```python
from build123d import *

# Parameters (mm, degrees)
F1_DEPTH = 3.5
F2_R     = 1.6
F3_DEPTH = 3.501


with BuildPart() as f1:
    # F0 (on Top) → F1 (new body)
    with BuildSketch(Plane.XY):
        with BuildLine():
            ThreePointArc((20, 4), (16, 0), (20, -4))
            Line((20, -4), (20, 4))
        make_face()
        with BuildLine():
            Line((-20, -4), (20, -4))
            ThreePointArc((20, -4), (16, 0), (20, 4))
            Line((20, 4), (-20, 4))
            ThreePointArc((-20, 4), (-17.1715728753, 2.8284271247), (-16, 0))
            ThreePointArc((-16, 0), (-17.1715728753, -2.8284271247), (-20, -4))
        make_face()
        with BuildLine():
            Line((20, 4), (20, -4))
            ThreePointArc((20, -4), (22.8284271247, -2.8284271247), (24, 0))
            ThreePointArc((24, 0), (22.8284271247, 2.8284271247), (20, 4))
        make_face()
        with BuildLine():
            ThreePointArc((-20, 4), (-24, 0), (-20, -4))
            Line((-20, -4), (-20, 4))
        make_face()
        with BuildLine():
            Line((-20, 4), (-20, -4))
            ThreePointArc((-20, -4), (-17.1715728753, -2.8284271247), (-16, 0))
            ThreePointArc((-16, 0), (-17.1715728753, 2.8284271247), (-20, 4))
        make_face()
    extrude(amount=F1_DEPTH)

    # F2 (on face) → F3 (cut, through all)
    with BuildSketch(Plane.XY.offset(3.5)):
        with BuildLine():
            ThreePointArc((-20, 1.6), (-21.6, 0), (-20, -1.6))
            Line((-20, -1.6), (-20, 1.6))
        make_face()
        with BuildLine():
            Line((-20, 1.6), (-20, -1.6))
            ThreePointArc((-20, -1.6), (-18.8686291501, -1.1313708499), (-18.4, 0))
            ThreePointArc((-18.4, 0), (-18.8686291501, 1.1313708499), (-20, 1.6))
        make_face()
        with BuildLine():
            ThreePointArc((20, 1.6), (18.4, 0), (20, -1.6))
            Line((20, -1.6), (20, 1.6))
        make_face()
        with BuildLine():
            Line((20, 1.6), (20, -1.6))
            ThreePointArc((20, -1.6), (21.1313708499, -1.1313708499), (21.6, 0))
            ThreePointArc((21.6, 0), (21.1313708499, 1.1313708499), (20, 1.6))
        make_face()
        with Locations((11.275196448, 0)):
            Circle(F2_R)
    extrude(amount=-F3_DEPTH, mode=Mode.SUBTRACT)


solid = f1.part
```
Build history of the part. All positions in model axes, mm. Round coordinates to 2 decimals unless told otherwise and drop trailing zeros. Write each loop counter-clockwise with the first axis right and the second up, starting at its lowest first coordinate (ties: lowest second). Pieces come first, ordered by that corner, then holes.
1) Band-saw the part on B-B, the plane x = 11. List the corners of the cut face in (y, z), and give its area (3 significant figures).
2) Mould opens along X. For faces 1 (the cylindrical face through (12.8, 0.48, 1.77)), 2 (the flat face through (0, 0, 0)), 3 (the cylindrical face through (-24, 0, 2)) say: +X half, -X half, draft (parallel to the pull), parting line (faces both ways), or undercut.
3) Band-saw the part on C-C, the plane y = -2.75. List the corners of the cut face in (x, z), and give its area (3 significant figures).
4) Band-saw the part on A-A, the plane z = 2.35. List the corners of the cut face in (x, y).
5) Drill centre lines: probe 1 along X at (y, z) = (1, 2.1); probe 2 along Y at (x, z) = (20, 1.35); probe 3 along X at (y, z) = (-0.5, 1.2). Where is each one in solid material? Low to high.
6) Pin check, flat tip, straight feed: pin 1 (1.9 mm diameter, centred on x = 11.28, y = 0, fed in from +Z). Stop position of the tip, or through.
Ans:
1. outline: (-4, 0) - (-1.58, 0) - (-1.58, 3.5) - (-4, 3.5) - close; (1.58, 0) - (4, 0) - (4, 3.5) - (1.58, 3.5) - close
1. area: 17.0 mm2
2. face 1: undercut
2. face 2: draft
2. face 3: -X half
3. outline: (-22.9, 0) - (22.9, 0) - (22.9, 3.5) - (-22.9, 3.5) - close
3. area: 160 mm2
4. outline: (-20, -4) - (20, -4) arc R4 ccw to (20, 4) - (-20, 4) arc R4 ccw to start; hole circle Ø3.2 at (-20, 0); hole circle Ø3.2 at (11.28, 0); hole circle Ø3.2 at (20, 0)
5. probe 1: x = -23.87 to -21.25, -18.75 to 10.03, 12.52 to 18.75, 21.25 to 23.87
5. probe 2: y = -4 to -1.6, 1.6 to 4
5. probe 3: x = -23.97 to -21.52, -18.48 to 9.76, 12.8 to 18.48, 21.52 to 23.97
6. pin 1: passes through
